The model under review builds one solid part; all positions refer to its coordinate system, in mm. Coordinates: 2 decimals unless noted, no trailing zeros. Order: outer loops, then holes, each group sorted by start corner. A loop starts at its lowest first (then second) coordinate and runs counter-clockwise, first axis right, second up. Notation, with made-up numbers: (19, 22.5) -> (34, 22.5) arc R27 cw to (34, 51.5) -> close; hole circle Ø7 at (55.25, 80). An arc over 180 degrees is marked (long way). Use one line per item in the form item = value.
from build123d import *

# Parameters (mm, degrees)
F0_W     = 65.160498
F0_H     = 46.986484
F1_DEPTH = 25.4
F3_D     = 17.78
F5_D     = 12.7
F7_D     = 12.7


with BuildPart() as f1:
    # F0 (on Front) → F1 (new body)
    with BuildSketch(Plane.XZ):
        Rectangle(F0_W, F0_H)
    extrude(amount=F1_DEPTH)

    # F3 (through all)
    with Locations(Plane.XZ.offset(25.4)):
        with Locations((0, 0)):
            Hole(F3_D / 2)

    # F5 (through all)
    with Locations(Plane.XY.offset(23.493242)):
        with Locations((-17.730748, -12.7)):
            Hole(F5_D / 2)

    # F7 (through all)
    with Locations(Plane.XY.offset(23.493242)):
        with Locations((19.28219, -12.7)):
            Hole(F7_D / 2)


solid = f1.part
Item 1: Clearance check with a flat-ended pin moving along its axis: pin 1 (14 mm diameter, centred on x = 0, z = 0, fed in from +Y). State where the tip first meets the part, or that it passes through.
Results found:
pin_1 = through
Item 2: To check wall thickness, follow L1, parallel to X at y = -7.25, z = -4; L2, parallel to Z at x = 0, y = -19; L3, parallel to X at y = -11, z = 19. State the ranges of each line that lie inside material, in increasing order. Write a range as from..to.
Results found:
L1 = -32.58..-20.99, -14.47..-7.94, 7.94..16.02, 22.54..32.58
L2 = -23.49..-8.89, 8.89..23.49
L3 = -32.58..-23.85, -11.61..13.16, 25.4..32.58
Item 3: We need section D-D (z = -12). Write out the cut boundary in (x, y), plus the area to 3 significant figures.
Results found:
outline = (-32.58, -25.4) -> (32.58, -25.4) -> (32.58, 0) -> (-32.58, 0) -> close; hole circle Ø12.7 at (-17.73, -12.7); hole circle Ø12.7 at (19.28, -12.7)
area = 1,400 mm²
Item 4: We need section C-C (x = 0). Write out the cut boundary in (y, z).
Results found:
outline = (-25.4, -23.49) -> (0, -23.49) -> (0, -8.89) -> (-25.4, -8.89) -> close; (-25.4, 8.89) -> (0, 8.89) -> (0, 23.49) -> (-25.4, 23.49) -> close
Item 5: We need section A-A (y = -12.7). Write out the cut boundary in (x, z).
Results found:
outline = (-32.58, -23.49) -> (-24.08, -23.49) -> (-24.08, 23.49) -> (-32.58, 23.49) -> close; (-11.38, -23.49) -> (12.93, -23.49) -> (12.93, 23.49) -> (-11.38, 23.49) -> close; (25.63, -23.49) -> (32.58, -23.49) -> (32.58, 23.49) -> (25.63, 23.49) -> close; hole circle Ø17.78 at (0, 0)
Item 6: We need section B-B (z = 0). Write out the cut boundary in (x, y), plus the area to 3 significant figures.
Results found:
outline = (-32.58, -25.4) -> (-8.89, -25.4) -> (-8.89, 0) -> (-32.58, 0) -> close; (8.89, -25.4) -> (32.58, -25.4) -> (32.58, 0) -> (8.89, 0) -> close; hole circle Ø12.7 at (-17.73, -12.7); hole circle Ø12.7 at (19.28, -12.7)
area = 950 mm²
Item 7: Draft analysis for pull direction X (two halves, no side actions). For faces 1 (the face through (1.93, -12.52, -8.68)), 2 (the face through (-32.58, -13, 0)), 3 (the face through (32.58, -13, 0)), state which applies: released by +X, released by -X, zero draft, split by the parting line, or undercut.
Results found:
face_1 = undercut
face_2 = released by -X
face_3 = released by +X
